Here's how the part is built. I have some questions about the finished solid (model axes, mm). Coordinates: 2 decimals unless noted, no trailing zeros. Write each loop counter-clockwise with the first axis right and the second up, starting at its lowest first coordinate (ties: lowest second). Pieces come first, ordered by that corner, then holes. Notation, with made-up numbers: (-21, -9) -> (17, -9) arc R10 ccw to (17, -2) -> close; hole circle Ø8 at (-1, 6.25). An arc over 180 degrees is marked (long way). Put each result on its own line as item: value.
```python
from build123d import *

# Parameters (mm, degrees)
SKETCH1_W           = 221.742
SKETCH1_H           = 139.7
SKETCH1_W_2         = 14.478
SKETCH1_H_2         = 65.278
BOSS_EXTRUDE3_DEPTH = 3.175
SKETCH3_R           = 2.032
CUT_EXTRUDE2_DEPTH  = 4.175
SKETCH4_R           = 2.032
CUT_EXTRUDE3_DEPTH  = 4.175
SKETCH5_R           = 2.54
CUT_EXTRUDE4_DEPTH  = 4.175


with BuildPart() as part:
    # Sketch1 → Boss-Extrude3 (new body)
    with BuildSketch(Plane.XY):
        with Locations((-110.871, 69.85)):
            Rectangle(SKETCH1_W, SKETCH1_H)
        with Locations((-228.981, 65.151)):
            Rectangle(SKETCH1_W_2, SKETCH1_H_2)
    extrude(amount=BOSS_EXTRUDE3_DEPTH)

    # Sketch3 → Cut-Extrude2 (cut, through all)
    with BuildSketch(Plane(origin=(0, 0, 0), x_dir=(-1, 0, 0), z_dir=(0, 0, -1))):
        with Locations((227.680130405, 80.681331583)):
            Circle(SKETCH3_R)
        with Locations((227.680130405, 48.931331583)):
            Circle(SKETCH3_R)
    extrude(amount=-CUT_EXTRUDE2_DEPTH, mode=Mode.SUBTRACT)

    # Sketch4 → Cut-Extrude3 (cut, through all)
    with BuildSketch(Plane.XY.offset(3.175)):
        with Locations((-17, 133.2)):
            Circle(SKETCH4_R)
    extrude(amount=-CUT_EXTRUDE3_DEPTH, mode=Mode.SUBTRACT)

    # Sketch5 → Cut-Extrude4 (cut, through all)
    with BuildSketch(Plane.XY.offset(3.175)):
        with Locations((-101.6, 69.85)):
            Circle(SKETCH5_R)
        with Locations((-12.7, 69.85)):
            Circle(SKETCH5_R)
    extrude(amount=-CUT_EXTRUDE4_DEPTH, mode=Mode.SUBTRACT)


solid = part.part
```
Item 1: If we mould it in two halves opening along Y, with no side actions, what happens to faces 1 (the cylindrical face through (-100.428, 67.597, 1.61)), 2 (the flat face through (-120, 71, 0))? For each: released by +Y, released by -Y, zero draft, split by the parting line, or undercut.
Output:
face 1: undercut
face 2: zero draft
Item 2: For P1, Ø6, axis at x = -12.7, y = 69.85, coming from the -Z side; P2, Ø1, axis at y = 127, z = 1.5, coming from the -X side; P3, Ø1, axis at x = -225.5, z = 1.5, coming from the -Y side; P4, Ø1, axis at x = -231, z = 2, coming from the +Y side, each with a flat end and sliding along its axis, tell me the tip position at first contact or that it passes through.
Output:
P1: stops at z = 0
P2: stops at x = -221.74
P3: stops at y = 32.51
P4: stops at y = 97.79
Item 3: Imagine slicing it at C-C on y = 113.5. Write out the boundary of the cut face in (x, z) (3 decimals), then the cut area to 3 significant figures.
Output:
outline: (-221.742, 0) -> (0, 0) -> (0, 3.175) -> (-221.742, 3.175) -> close
area: 704 mm²
Item 4: Please list where these lines run through material, in increasing order: line 1 along Y through (x, z) = (-17, 0.8); line 2 along X through (y, z) = (69, 2.3); line 3 along X through (y, z) = (68.5, 2.3). Write a range as from..to.
Output:
line 1: y = 0..131.17, 135.23..139.7
line 2: x = -236.22..-103.99, -99.21..-15.09, -10.31..0
line 3: x = -236.22..-103.75, -99.45..-14.85, -10.55..0
Item 5: Imagine slicing it at B-B on x = -12.7. Write out the boundary of the cut face in (y, z) (3 decimals), then the cut area to 3 significant figures.
Output:
outline: (0, 0) -> (67.31, 0) -> (67.31, 3.175) -> (0, 3.175) -> close; (72.39, 0) -> (139.7, 0) -> (139.7, 3.175) -> (72.39, 3.175) -> close
area: 427 mm²
Item 6: Imagine slicing it at A-A on y = 69.85. Write out the boundary of the cut face in (x, z) (3 decimals).
Output:
outline: (-236.22, 0) -> (-104.14, 0) -> (-104.14, 3.175) -> (-236.22, 3.175) -> close; (-99.06, 0) -> (-15.24, 0) -> (-15.24, 3.175) -> (-99.06, 3.175) -> close; (-10.16, 0) -> (0, 0) -> (0, 3.175) -> (-10.16, 3.175) -> close
